Autodesk Inventor part; units mm, degrees
ref_plane "YZ Plane" through (0, 0, 0) normal (1, 0, 0) x (0, 1, 0)
ref_plane "XZ Plane" through (0, 0, 0) normal (0, 1, 0) x (-1, 0, 0)
ref_plane "XY Plane" through (0, 0, 0) normal (0, 0, 1) x (1, 0, 0)
sketch "Sketch6" plane through (0, 0, 0) normal (0, 1, 0) x (-1, 0, 0)
  line L0 (315, -990) -> (-315, -990)
  line L1 (-315, -990) -> (-315, 990)
  line L2 (-315, 990) -> (315, 990)
  line L3 (315, 990) -> (315, -990)
  line L4 (315, -990) -> (-315, 990) construction
  line L5 (-315, -990) -> (315, 990) construction
  point P0 (0, 0)
  dimension "d52" = 630
  dimension "d53" = 1980
extrude "Plate2" add sketch "Sketch6" along normal blind 0.5
sketch "Sketch11" plane through (314.5, 0, -990) normal (1, 0, 0) x (0, 1, 0)
  line L0 (0, 1980) -> (0, 0)
  line L1 (0, 0) -> (10, 0)
  line L2 (10, 0) -> (10, 1980)
  line L3 (10, 1980) -> (0, 1980)
edge flange "Flange2" height 10 angle 90 thickness 0.5 bend radius 0.5 thickness toward (1, 0, 0) relief tear relief width 0.5 relief depth 0.25 edges at (315, 0.5, 0) wall of the first edge with corners at (314.5, 0, 990) (314.5, 0, -990) (314.5, 10, -990) (314.5, 10, 990)
bend "Bend3"
corner "Corner3"
sketch "Sketch12" plane through (315, 9.5, -990) normal (0, 1, 0) x (-1, 0, 0)
  line L0 (0, 1980) -> (0, 0)
  line L1 (0, 0) -> (10, 0)
  line L2 (10, 0) -> (10, 1980)
  line L3 (10, 1980) -> (0, 1980)
edge flange "Flange3" height 10 angle 90 thickness 0.5 bend radius 0.5 thickness toward (0, 1, 0) relief tear relief width 0.5 relief depth 0.25 edges at (314.5, 10, 0) wall of the first edge with corners at (315, 9.5, 990) (315, 9.5, -990) (305, 9.5, -990) (305, 9.5, 990)
bend "Bend4"
corner "Corner4"
sketch "Sketch13" plane through (-314.5, 0, 990) normal (-1, 0, 0) x (0, -1, 0)
  line L0 (0, -1980) -> (0, 0)
  line L1 (0, 0) -> (-10, 0)
  line L2 (-10, 0) -> (-10, -1980)
  line L3 (-10, -1980) -> (0, -1980)
edge flange "Flange4" height 10 angle 90 thickness 0.5 bend radius 0.5 thickness toward (-1, 0, 0) relief tear relief width 0.5 relief depth 0.25 edges at (-315, 0.5, 0) wall of the first edge with corners at (-314.5, 0, -990) (-314.5, 0, 990) (-314.5, 10, 990) (-314.5, 10, -990)
bend "Bend5"
corner "Corner5"
sketch "Sketch14" plane through (-315, 9.5, 990) normal (0, 1, 0) x (-1, 0, 0)
  line L0 (0, -1980) -> (0, 0)
  line L1 (0, 0) -> (-10, 0)
  line L2 (-10, 0) -> (-10, -1980)
  line L3 (-10, -1980) -> (0, -1980)
edge flange "Flange5" height 10 angle 90 thickness 0.5 bend radius 0.5 thickness toward (0, 1, 0) relief tear relief width 0.5 relief depth 0.25 edges at (-314.5, 10, 0) wall of the first edge with corners at (-315, 9.5, -990) (-315, 9.5, 990) (-305, 9.5, 990) (-305, 9.5, -990)
bend "Bend6"
corner "Corner6"
equation "\"d53\" = ЖАБРЫ_базовая_длина_дл_лист"
equation "\"d54\" = Thickness"
equation "\"d84\" = BendReliefWidth"
equation "\"d85\" = BendReliefDepth"
equation "\"d86\" = MinimumRemnant"
equation "\"d87\" = TransitionRadius"
equation "\"d90\" = BendRadius"
equation "\"d91\" = CornerReliefSize"
equation "\"d92\" = GapSize"
equation "\"d93\" = JacobiRadiusSize"
equation "\"d94\" = BendReliefWidth"
equation "\"d95\" = BendReliefDepth"
equation "\"d96\" = MinimumRemnant"
equation "\"d97\" = TransitionRadius"
equation "\"d100\" = BendRadius"
equation "\"d101\" = CornerReliefSize"
equation "\"d102\" = GapSize"
equation "\"d103\" = JacobiRadiusSize"
equation "\"d104\" = BendReliefWidth"
equation "\"d105\" = BendReliefDepth"
equation "\"d106\" = MinimumRemnant"
equation "\"d107\" = TransitionRadius"
equation "\"d110\" = BendRadius"
equation "\"d111\" = CornerReliefSize"
equation "\"d112\" = GapSize"
equation "\"d113\" = JacobiRadiusSize"
equation "\"d114\" = BendReliefWidth"
equation "\"d115\" = BendReliefDepth"
equation "\"d116\" = MinimumRemnant"
equation "\"d117\" = TransitionRadius"
equation "\"d120\" = BendRadius"
equation "\"d121\" = CornerReliefSize"
equation "\"d122\" = GapSize"
equation "\"d123\" = JacobiRadiusSize"
equation "\"BendRadius\" = Thickness"
equation "\"BendReliefWidth\" = Thickness"
equation "\"BendReliefDepth\" = 0.5 * Thickness"
equation "\"CornerReliefSize\" = 4 * Thickness"
equation "\"MinimumRemnant\" = 2 * Thickness"
equation "\"TransitionRadius\" = BendRadius"
equation "\"JacobiRadiusSize\" = BendRadius"
equation "\"GapSize\" = Thickness"
properties part number "MSC 808 sheet gills" material "Stainless Steel"
Here's how the part is built. I have some questions about the finished solid (model axes, mm). Coordinates: 2 decimals unless noted, no trailing zeros. Order: outer loops, then holes, each group sorted by start corner. A loop starts at its lowest first (then second) coordinate and runs counter-clockwise, first axis right, second up. Notation, with made-up numbers: (-34, 17) - (-21, 17) arc R29 ccw to (-21, 42) - close; hole circle Ø9 at (82.25, 66). An arc over 180 degrees is marked (long way). Use CSV: the item, a comma, the result in double quotes. Start each with the question number.
1. Please list where these lines run through material, in increasing order: line 1 (X direction, y = 5.5, z = 341.5); line 2 (Y direction, x = -128, z = -752). Write a range as from..to.
2. Suppose I cut it at A-A on z = -161.5. List the corners of the cut face in (x, y) for me, then the cut area to 3 significant figures.
3. Suppose I cut it at B-B on y = 6. List the corners of the cut face in (x, z) for me.
4. Suppose I cut it at C-C on x = -165.5. List the corners of the cut face in (y, z) for me.
Output:
1,line 1,"x = -315..-314.5, 314.5..315"
1,line 2,"y = 0..0.5"
2,outline,"(-315, 1) arc R1 ccw to (-314, 0) - (314, 0) arc R1 ccw to (315, 1) - (315, 9) arc R1 ccw to (314, 10) - (305, 10) - (305, 9.5) - (314, 9.5) arc R0.5 cw to (314.5, 9) - (314.5, 1) arc R0.5 cw to (314, 0.5) - (-314, 0.5) arc R0.5 cw to (-314.5, 1) - (-314.5, 9) arc R0.5 cw to (-314, 9.5) - (-305, 9.5) - (-305, 10) - (-314, 10) arc R1 ccw to (-315, 9) - close"
2,area,"333 mm2"
3,outline,"(-315, -990) - (-314.5, -990) - (-314.5, 990) - (-315, 990) - close; (314.5, -990) - (315, -990) - (315, 990) - (314.5, 990) - close"
4,outline,"(0, -990) - (0.5, -990) - (0.5, 990) - (0, 990) - close"
